Design review of the part built by this model. Coordinates are the model's own, in mm. A direction names the side the tool comes from. Coordinates: 2 decimals unless noted, no trailing zeros. Loops run counter-clockwise (first coordinate to the right, second up) from the corner with the lowest first, then second, coordinate; pieces in that order, holes last. Notation, with made-up numbers: (19, 77.5) - (31, 77.5) arc R30 ccw to (31, 112.5) - close; hole circle Ø8 at (63, 88.25). An arc over 180 degrees is marked (long way). Answer in a Markdown table with one row per item. Add a question column.
(1) We need section C-C, the plane y = 5.5. Write out the cut boundary in (x, z).
(2) To check wall thickness, follow L1, parallel to Y at x = 0, z = 1.35; L2, parallel to Y at x = -5.25, z = 3.35; L3, parallel to Y at x = 5.75, z = 2.8. State the ranges of each line that lie inside material, in increasing order. Write a range as [from, to].
(3) We need section D-D, the plane x = 4.25. Write out the cut boundary in (y, z).
(4) We need section B-B, the plane x = 1. Write out the cut boundary in (y, z).
(5) We need section A-A, the plane y = 0.5. Write out the cut boundary in (x, z), plus the area to 3 significant figures.
(6) The part is to be moulded in two halves that separate along Y. For faces 1 (the face through (0.56, -6.12, 1.97)), 2 (the face through (2.84, 5.423, 1.972)), 3 (the face through (6.12, 0.56, 1.97)), say which applies: released by +Y, released by -Y, zero draft, split by the parting line, or undercut.
(7) For faces 4 (the face through (1.826, -5.843, 1.972)), 5 (the face through (-2.86, 5.44, 1.97)), 6 (the face through (6.1, -0.55, 1.97)), list the 3-axis set-ups (+Z, -Z, +X, -X, +Y, -Y) from which the entire face can be reached by the end or side of a thin tool; tool diameter is ignored.
(8) Clearance check with flat-ended pins moving along their axes: pin 1 (2 mm diameter, centred on y = 4.5, z = 3.5, fed in from -X); pin 2 (1 mm diameter, centred on x = 0, z = 0.5, fed in from -Y); pin 3 (1.5 mm diameter, centred on y = 2, z = 3.5, fed in from +X). State where each tip first meets the part, or that it passes through.
from build123d import *

# Parameters (mm, degrees)
SKETCH1_R           = 7
SKETCH1_R_2         = 1.5
BOSS_EXTRUDE1_DEPTH = 4
CUT_EXTRUDE2_DEPTH  = 5
CIRPATTERN2_COUNT   = 16


with BuildPart() as part:
    # Sketch1 → Boss-Extrude1 (new body)
    with BuildSketch(Plane.XY):
        Circle(SKETCH1_R)
        Circle(SKETCH1_R_2, mode=Mode.SUBTRACT)
    extrude(amount=BOSS_EXTRUDE1_DEPTH)

    # Sketch4 → Cut-Extrude2 (cut, through all)
    with BuildSketch(Plane.XY):
        with BuildLine():
            ThreePointArc((-0.144865992, 4.997900944), (0, 5), (0.144865992, 4.997900944))
            ThreePointArc((0.144865992, 4.997900944), (0.250687134, 5.037371727), (0.298978368, 5.139469785))
            ThreePointArc((0.298978368, 5.139469785), (0.554893378, 6.109748451), (1.171724109, 6.90123631))
            ThreePointArc((1.171724109, 6.90123631), (0, 7), (-1.171724109, 6.90123631))
            ThreePointArc((-1.171724109, 6.90123631), (-0.554893378, 6.109748451), (-0.298978368, 5.139469785))
            ThreePointArc((-0.298978368, 5.139469785), (-0.250687134, 5.037371727), (-0.144865992, 4.997900944))
        make_face()
    cut_extrude2 = extrude(amount=CUT_EXTRUDE2_DEPTH, mode=Mode.SUBTRACT)

    # CirPattern2: Cut-Extrude2 ×16 about axis
    cirpattern2_axis = Axis((0, 0, 0), (0, 0, 1))
    for i in range(1, CIRPATTERN2_COUNT):
        add(cut_extrude2.rotate(cirpattern2_axis, i * 360 / CIRPATTERN2_COUNT), mode=Mode.SUBTRACT)


solid = part.part
Responses:
| question | item | result |
|---|---|---|
| 1 | outline | (-4.06, 0) - (-2.93, 0) - (-2.93, 4) - (-4.06, 4) - close; (-1.82, 0) - (-0.35, 0) - (-0.35, 4) - (-1.82, 4) - close; (0.35, 0) - (1.82, 0) - (1.82, 4) - (0.35, 4) - close; (2.93, 0) - (4.06, 0) - (4.06, 4) - (2.93, 4) - close |
| 2 | L1 | y = [-5, -1.5], [1.5, 5] |
| 2 | L2 | y = [-4.05, -2.66], [-1.79, -0.31], [0.31, 1.79], [2.66, 4.05] |
| 2 | L3 | y = [-3.99, -3.31], [-1.83, -0.41], [0.41, 1.83], [3.31, 3.99] |
| 3 | outline | (-3.72, 0) - (3.72, 0) - (3.72, 4) - (-3.72, 4) - close |
| 4 | outline | (-6.74, 0) - (-1.12, 0) - (-1.12, 4) - (-6.74, 4) - close; (1.12, 0) - (6.74, 0) - (6.74, 4) - (1.12, 4) - close |
| 5 | outline | (-5.99, 0) - (-1.41, 0) - (-1.41, 4) - (-5.99, 4) - close; (1.41, 0) - (5.99, 0) - (5.99, 4) - (1.41, 4) - close |
| 5 | area | 36.6 mm2 |
| 6 | face 1 | released by -Y |
| 6 | face 2 | released by +Y |
| 6 | face 3 | undercut |
| 7 | face 4 | +Z, -Z |
| 7 | face 5 | +Z, -Z, +Y |
| 7 | face 6 | +Z, -Z, +X |
| 8 | pin 1 | stops at x = -5.93 |
| 8 | pin 2 | stops at y = -5.99 |
| 8 | pin 3 | stops at x = 6.89 |
